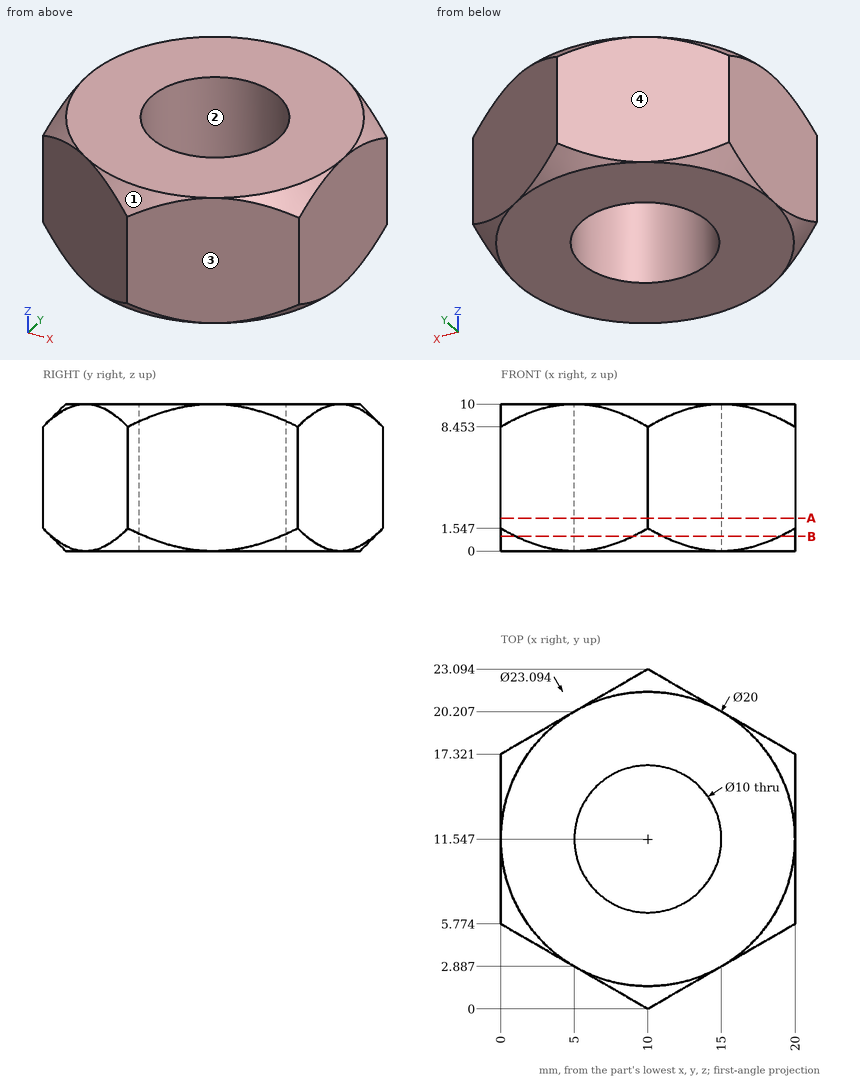
Source: three-view drawing plus pictorial views. Frame: mm from the lowest corner of the part. Round coordinates to 2 decimals unless told otherwise and drop trailing zeros. Loops run counter-clockwise (first coordinate to the right, second up) from the corner with the lowest first, then second, coordinate; pieces in that order, holes last. Notation, with made-up numbers: M -4,57.25 L 2,57.25 A17 cw 2,85.25 Z; hole C 27,44 d4. An arc over 180 degrees is marked long. Put each result on its own line as item: value. Start each with the question number.
(1) Material intervals for line 1 along X through (y, z) = (7.5, 4.75) (1 decimal); line 2 along X through (y, z) = (11, 4.25); line 3 along Y through (x, z) = (9.5, 0.75) (1 decimal), sorted ascending. Write a range as [from, to].
(2) Section query A-A (z = 2.25). Return loops of the section in (x, y) (1 decimal).
(3) Contact query for flat-ended pins moving along their axis: pin 1 Ø1 at (x, z) = (5.5, 1.5) entering from -Y; pin 2 Ø4 at (x, z) = (14.5, 5.5) entering from +Y. Output: stop coordinate, or through.
(4) Draft query along X for the marked faces 1, 2, 3 and 4. Return one class per face: +X half, -X half, draft (parallel to the pull), parting line (faces both ways), or undercut.
(5) Section query B-B (z = 1). Return loops of the section in (x, y) (1 decimal).
Findings below:
1. line 1: x = [0, 7.1], [12.9, 20]
1. line 2: x = [0, 5.03], [14.97, 20]
1. line 3: y = [0.8, 6.6], [16.5, 22.3]
2. outline: M 0,5.8 L 10,0 L 20,5.8 L 20,17.3 L 10,23.1 L 0,17.3 Z; hole C 10,11.5 d10
3. pin 1: stops at y = 2.31
3. pin 2: stops at y = 21.65
4. face 1: parting line
4. face 2: undercut
4. face 3: +X half
4. face 4: -X half
5. outline: M 0,7 A11 ccw 1,5.2 L 9,0.6 A11 ccw 11,0.6 L 19,5.2 A11 ccw 20,7 L 20,16.1 A11 ccw 19,17.9 L 11,22.5 A11 ccw 9,22.5 L 1,17.9 A11 ccw 0,16.1 Z; hole C 10,11.5 d10
